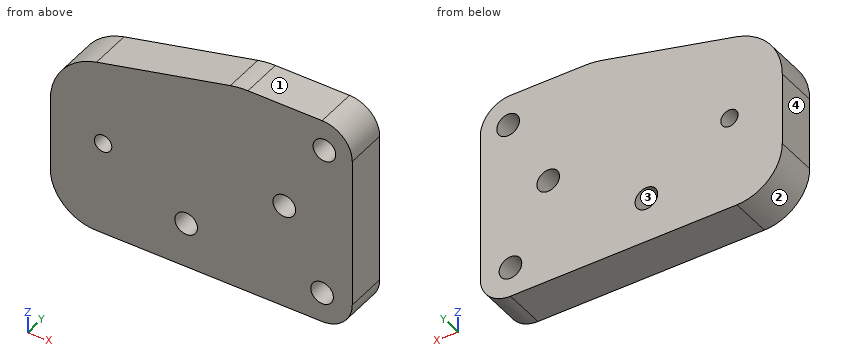
from build123d import *

# Parameters (mm, degrees)
SKETCH1_R           = 1.5
SKETCH1_R_2         = 1.15
BOSS_EXTRUDE1_DEPTH = 5.5
FILLET1_R           = 6
FILLET2_R           = 8
FILLET3_R           = 4
FILLET4_R           = 4
FILLET5_R           = 10


with BuildPart() as part:
    # Sketch1 → Boss-Extrude1 (new body)
    with BuildSketch(Plane(origin=(0, 0, 0), x_dir=(1, 0, 0), z_dir=(0, 1, 0))):
        Polygon((0, 16), (25, 10), (40, 10), (40, 38), (0, 38), align=None)
        with Locations(Location((36, 34, 0), (0, 0, 270))):
            Circle(SKETCH1_R, mode=Mode.SUBTRACT)
        with Locations(Location((36.311245585, 14, 0), (0, 0, 270))):
            Circle(SKETCH1_R, mode=Mode.SUBTRACT)
        with Locations(Location((31, 24, 0), (0, 0, 270))):
            Circle(SKETCH1_R, mode=Mode.SUBTRACT)
        with Locations(Location((18, 32, 0), (0, 0, 270))):
            Circle(SKETCH1_R, mode=Mode.SUBTRACT)
        with Locations(Location((7, 25.5, 0), (0, 0, 270))):
            Circle(SKETCH1_R_2, mode=Mode.SUBTRACT)
    extrude(amount=BOSS_EXTRUDE1_DEPTH)

    # Fillet1
    fillet1_edges = [part.edges().sort_by_distance(p)[0] for p in [
        (0, 2.75, -38),
    ]]
    fillet(fillet1_edges, radius=FILLET1_R)

    # Fillet2
    fillet2_edges = [part.edges().sort_by_distance(p)[0] for p in [
        (0, 2.75, -16),
    ]]
    fillet(fillet2_edges, radius=FILLET2_R)

    # Fillet3
    fillet3_edges = [part.edges().sort_by_distance(p)[0] for p in [
        (40, 2.75, -38),
    ]]
    fillet(fillet3_edges, radius=FILLET3_R)

    # Fillet4
    fillet4_edges = [part.edges().sort_by_distance(p)[0] for p in [
        (40, 2.75, -10),
    ]]
    fillet(fillet4_edges, radius=FILLET4_R)

    # Fillet5
    fillet5_edges = [part.edges().sort_by_distance(p)[0] for p in [
        (25, 2.75, -10),
    ]]
    fillet(fillet5_edges, radius=FILLET5_R)


solid = part.part
Design review of the part built by this model. Coordinates are the model's own, in mm. Face numbers are marked on the shaded views. Coordinates: 2 decimals unless noted, no trailing zeros. Loops run counter-clockwise (first coordinate to the right, second up) from the corner with the lowest first, then second, coordinate; pieces in that order, holes last.
Item 1: Wall thickness on L1, parallel to X at y = 1.7, z = -32; L2, parallel to X at y = 5, z = -24.5; L3, parallel to X at y = 2.4, z = -25: over which ranges is each line inside the solid? List them lowest first.
Completed:
L1: x = 0 to 16.5, 19.5 to 40
L2: x = 0 to 6.43, 7.57 to 29.59, 32.41 to 40
L3: x = 0 to 5.96, 8.04 to 29.88, 32.12 to 40
Item 2: Draft analysis for pull direction Z (two halves, no side actions). For the marked faces 1, 2, 3 and 4, state which applies: pulls with the +Z half, pulls with the -Z half, needs draft (parallel to the pull), parting line crosses it, or undercut.
Completed:
face 1: pulls with the +Z half
face 2: pulls with the -Z half
face 3: undercut
face 4: needs draft
Item 3: Add section B-B (y = 3). Write out the cut boundary in (x, z), and give its area (3 significant figures).
Completed:
outline: (0, -32) arc R6 ccw to (6, -38) - (36, -38) arc R4 ccw to (40, -34) - (40, -14) arc R4 ccw to (36, -10) - (26.18, -10) arc R10 ccw to (23.85, -10.28) - (6.13, -14.53) arc R8 ccw to (0, -22.31) - close; hole circle Ø2.3 at (7, -25.5); hole circle Ø3 at (18, -32); hole circle Ø3 at (31, -24); hole circle Ø3 at (36, -34); hole circle Ø3 at (36.31, -14)
area: 990 mm2
Item 4: Add section A-A (x = 31). Write out the cut boundary in (y, z), and give its area (4 significant figures).
Completed:
outline: (0, -38) - (5.5, -38) - (5.5, -25.5) - (0, -25.5) - close; (0, -22.5) - (5.5, -22.5) - (5.5, -10) - (0, -10) - close
area: 137.5 mm2
Item 5: Clearance check with flat-ended pins moving along their axes: pin 1 (2.5 mm diameter, centred on x = 36, z = -34, fed in from -Y); pin 2 (6 mm diameter, centred on x = 21, z = -18, fed in from -Y). State where each tip first meets the part, or that it passes through.
Completed:
pin 1: passes through
pin 2: stops at y = 0
